Here's how the part is built. I have some questions about the finished solid (model axes, mm). Round coordinates to 2 decimals unless told otherwise and drop trailing zeros. Loops run counter-clockwise (first coordinate to the right, second up) from the corner with the lowest first, then second, coordinate; pieces in that order, holes last. Notation, with made-up numbers: M 57.5,76 L 65.5,76 A22 cw 65.5,114 Z; hole C -9,-29 d6. An arc over 180 degrees is marked long. Answer as CSV lines item,"result".
```python
from build123d import *

# Parameters (mm, degrees)
SKETCH1_W           = 12
SKETCH1_H           = 4
BOSS_EXTRUDE1_DEPTH = 12
SKETCH2_OUTSIDE_W   = 17.488
SKETCH2_OUTSIDE_H   = 17.488
SKETCH2_OUTSIDE_R   = 6
CUT_EXTRUDE1_DEPTH  = 12


with BuildPart() as part:
    # Sketch1 → Boss-Extrude1 (new body)
    with BuildSketch(Plane(origin=(0, 0, 0), x_dir=(1, 0, 0), z_dir=(0, 1, 0))):
        Rectangle(SKETCH1_W, SKETCH1_H)
    extrude(amount=BOSS_EXTRUDE1_DEPTH)

    # Sketch2 outside → Cut-Extrude1 (cut)
    with BuildSketch(Plane(origin=(0, 0, -2), x_dir=(-1, 0, 0), z_dir=(0, 0, -1))):
        with Locations((0, 6)):
            Rectangle(SKETCH2_OUTSIDE_W, SKETCH2_OUTSIDE_H)
        with Locations((0, 6)):
            Circle(SKETCH2_OUTSIDE_R, mode=Mode.SUBTRACT)
    extrude(amount=-CUT_EXTRUDE1_DEPTH, mode=Mode.SUBTRACT)

    # Sketch5 → Cut-Revolve1 (revolve, cut)
    with BuildSketch(Plane(origin=(0, 0, 0), x_dir=(0, 0, -1), z_dir=(1, 0, 0))):
        Polygon((0.663673358, 10.775), (1.327346716, 12), (0.663673358, 12), align=None)
    revolve(axis=Axis((0, 6, 0), (0, 0, -1)), mode=Mode.SUBTRACT)


solid = part.part
```
1. I want a section at A-A, the plane x = 0. Please give me the cut outline in (y, z) (3 decimals).
Evaluation:
outline,"M 0,-2 L 12,-2 L 12,-1.327 L 10.775,-0.664 L 12,-0.664 L 12,2 L 0,2 L 0,-0.664 L 1.225,-0.664 L 0,-1.327 Z"
2. If I drill on line 1 (Z direction, x = -5.5, y = 3.75); line 2 (Z direction, x = 5.25, y = 4.25); line 3 (X direction, y = 9.25, z = -0.05), over which ranges is the centre line in solid material (lowest first)? Write a range as [from, to].
Evaluation:
line 1,"z = [-2, -1.3], [-0.66, 2]"
line 2,"z = [-2, -1.07], [-0.66, 2]"
line 3,"x = [-5.04, 5.04]"
3. For P1, Ø1, axis at x = 4.5, z = 0.5, coming from the -Y side, with a flat end and sliding along its axis, tell me the tip position at first contact or that it passes through.
Evaluation:
P1,"stops at y = 1.53"
4. I want a section at B-B, the plane z = 0.7. Please give me the cut outline in (x, y).
Evaluation:
outline,"C 0,6 d12"
5. I want a section at C-C, the plane y = 6. Please give me the cut outline in (x, z) (3 decimals).
Evaluation:
outline,"M -6,-2 L 6,-2 L 6,-1.327 L 4.775,-0.664 L 6,-0.664 L 6,2 L -6,2 L -6,-0.664 L -4.775,-0.664 L -6,-1.327 Z"
